Geometry: final body of the model. Coordinates: model frame, mm. A direction names the side the tool comes from. Give positions to 0.01 mm unless a question says otherwise; leave off trailing zeros. Write each loop counter-clockwise with the first axis right and the second up, starting at its lowest first coordinate (ties: lowest second). Pieces come first, ordered by that corner, then holes. Notation, with made-up numbers: (-27, 69.25) -> (13, 69.25) arc R19 ccw to (13, 80.25) -> close; hole circle Ø4 at (76, 48). An arc over 180 degrees is marked (long way). Answer in a Markdown table with one row per item. Add a question column.
Item 1: Access query for faces 5 (the flat face through (27.8, 0, 0)), 6 (the flat face through (0.897, 1.293, 0.76)). Directions: +Z, -Z, +X, -X, +Y, -Y. A direction counts if a zero-diameter tool reaches every point of the face in a straight line with its end or side. Return the directions, or none.
Item 2: Draft query along Z for faces 1 (the conical face through (2.65, -0.25, -0.06)), 2 (the flat face through (2.8, -2, 2)), 3 (the cylindrical face through (14.88, -2.44, 0.54)), 4 (the flat face through (1, 0, 1.5)). Return one class per face: +Z half, -Z half, draft (parallel to the pull), parting line (faces both ways), or undercut.
Item 3: First-contact query: P1, Ø2, axis at x = 22.5, y = 0.5, coming from the -Z side; P2, Ø4, axis at x = 10, z = -2, coming from the -Y side; P3, Ø1.4, axis at x = 1, y = 0.5, coming from the -Z side. Flat tips, straight axial feed; report the tip coordinate or a pass-through.
Item 4: Section query A-A on x = 3.5. Output: boundary loops of the cut face in (y, z), plus the area to 3 significant figures.
Item 5: Material intervals for probe 1 along Y at (x, z) = (1.9, 0); probe 2 along Y at (x, z) = (9.5, -2); probe 3 along Z at (x, y) = (1.95, 0), sorted ascending. Write a range as from..to.
```python
from build123d import *

# Parameters (mm, degrees)
SKETCH_1_W                = 2.8
SKETCH_1_H                = 5
SKETCH_2_R                = 2.5
EXTRUDE_1_DEPTH           = 25
CUT_EXTRUDE_1_DEPTH       = 1.82
HOLE_WIZARD_3_0_3_1_D     = 3
HOLE_WIZARD_3_0_3_1_DEPTH = 0.113974596
HOLE_WIZARD_3_0_3_1_TIP   = 0.866025404
CHAMFER_1_SIZE            = 0.4905
FILLET_1_R                = 2.7


with BuildPart() as part:
    # Эскиз1 → Повернуть1 (revolve)
    with BuildSketch(Plane(origin=(0, 0, 0), x_dir=(-1, 0, 0), z_dir=(0, 0, -1))):
        with Locations((-1.4, 2.5)):
            Rectangle(SKETCH_1_W, SKETCH_1_H)
    revolve(axis=Axis((2.8, 0, 0), (-1, 0, 0)))

    # Эскиз2 → Бобышка-Вытянуть1 (add)
    with BuildSketch(Plane(origin=(2.8, 0, 0), x_dir=(0, 0, -1), z_dir=(1, 0, 0))):
        Circle(SKETCH_2_R)
    extrude(amount=EXTRUDE_1_DEPTH)

    # Эскиз3 → Вырез-Вытянуть1 (cut)
    with BuildSketch(Plane.ZY):
        Polygon((0, 1.732050808), (-1.5, 0.866025404), (-1.5, -0.866025404), (0, -1.732050808), (1.5, -0.866025404), (1.5, 0.866025404), align=None)
    extrude(amount=-CUT_EXTRUDE_1_DEPTH, mode=Mode.SUBTRACT)

    # Диаметр отверстия Ø3.0 (3)1
    with Locations(Plane.ZY.offset(-1.82)):
        with Locations((0, 0)):
            Hole(HOLE_WIZARD_3_0_3_1_D / 2, depth=HOLE_WIZARD_3_0_3_1_DEPTH)
            with Locations((0, 0, -(HOLE_WIZARD_3_0_3_1_DEPTH + HOLE_WIZARD_3_0_3_1_TIP / 2))):  # 120° drill point
                Cone(0, HOLE_WIZARD_3_0_3_1_D / 2, HOLE_WIZARD_3_0_3_1_TIP, mode=Mode.SUBTRACT)

    # Фаска1
    chamfer_1_edges = [part.edges().sort_by_distance(p)[0] for p in [
        (27.8, 0, 2.5),
    ]]
    chamfer(chamfer_1_edges, length=CHAMFER_1_SIZE)

    # Скругление1
    fillet_1_edges = [part.edges().sort_by_distance(p)[0] for p in [
        (0, -5, 0),
    ]]
    fillet(fillet_1_edges, radius=FILLET_1_R)


solid = part.part
```
Findings below:
| question | item | result |
|---|---|---|
| 1 | face 5 | +Z, -Z, +X, +Y, -Y |
| 1 | face 6 | -X |
| 2 | face 1 | undercut |
| 2 | face 2 | draft |
| 2 | face 3 | parting line |
| 2 | face 4 | undercut |
| 3 | P1 | stops at z = -2.5 |
| 3 | P2 | stops at y = -2.5 |
| 3 | P3 | stops at z = -4.79 |
| 4 | outline | circle Ø5 at (0, 0) |
| 4 | area | 19.6 mm^2 |
| 5 | probe 1 | y = -4.88..-1.5, 1.5..4.88 |
| 5 | probe 2 | y = -1.5..1.5 |
| 5 | probe 3 | z = -4.89..-1.47, 1.47..4.89 |
